Geometry: final body of the model. Coordinates: model frame, mm. Face numbers are marked on the shaded views. A direction names the side the tool comes from. Give positions to 0.01 mm unless a question says otherwise; leave off trailing zeros. Loops run counter-clockwise (first coordinate to the right, second up) from the corner with the lowest first, then second, coordinate; pieces in that order, holes last. Notation, with made-up numbers: (77.5, 44.5) -> (119.5, 44.5) arc R26 ccw to (119.5, 82.5) -> close; hole circle Ø7 at (23.5, 65). An arc over 180 degrees is marked (long way). Answer in a Markdown table with one row per item. Add a question column.
1) First-contact query: P1, Ø6, axis at x = -17.5, y = 18, coming from the +Z side; P2, Ø2, axis at y = -3, z = -0.5, coming from the +X side. Flat tips, straight axial feed; report the tip coordinate or a pass-through.
2) Section query D-D (x = 10). Return the cut outline in (y, z), plus the area to 3 significant figures.
3) Section query C-C (z = 1.25). Return the cut outline in (x, y).
4) Section query A-A (x = 0). Return the cut outline in (y, z).
5) Line query: line 1 (Z direction, x = 11, y = -19.5); line 2 (Z direction, x = 6.5, y = 1); line 3 (Y direction, x = 0, z = 2.5). Output: solid intervals per line, ascending. Write a range as from..to.
6) Access query for the marked faces 1 and 2. Directions: +Z, -Z, +X, -X, +Y, -Y. A direction counts if a zero-diameter tool reaches every point of the face in a straight line with its end or side. Return the directions, or none.
```python
from build123d import *

# Parameters (mm, degrees)
F0_R     = 25.4
F0_R_2   = 7.9375
F0_R_3   = 3.8735
F1_DEPTH = 1.5875
F2_DEPTH = 5.08
F3_SIZE  = 0.508
F4_DEPTH = 0.508


with BuildPart() as f1:
    # F0 (on Top) → F1 (new body)
    with BuildSketch(Plane.XY):
        Circle(F0_R)
        Circle(F0_R_2, mode=Mode.SUBTRACT)
        Circle(F0_R_2)
        Circle(F0_R_3, mode=Mode.SUBTRACT)
        Circle(F0_R_3)
    extrude(amount=-F1_DEPTH)

    # F0 (on Top) → F2 (join)
    with BuildSketch(Plane.XY):
        Circle(F0_R_3)
    extrude(amount=F2_DEPTH)

    # F3
    f3_edges = [f1.edges().sort_by_distance(p)[0] for p in [
        (-3.8735, 0, 5.08),
    ]]
    chamfer(f3_edges, length=F3_SIZE)

    # F0 (on Top) → F4 (join)
    with BuildSketch(Plane.XY):
        Circle(F0_R_2)
        Circle(F0_R_3, mode=Mode.SUBTRACT)
    extrude(amount=F4_DEPTH)


solid = f1.part
```
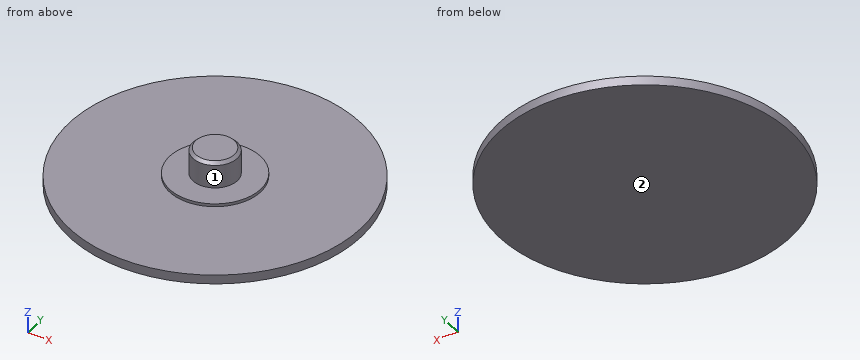
Evaluation:
| question | item | result |
|---|---|---|
| 1 | P1 | z = 0 |
| 1 | P2 | x = 25.32 |
| 2 | outline | (-23.35, -1.59) -> (23.35, -1.59) -> (23.35, 0) -> (-23.35, 0) -> close |
| 2 | area | 74.1 mm² |
| 3 | outline | circle Ø7.75 at (0, 0) |
| 4 | outline | (-25.4, -1.59) -> (25.4, -1.59) -> (25.4, 0) -> (7.94, 0) -> (7.94, 0.51) -> (3.87, 0.51) -> (3.87, 4.57) -> (3.37, 5.08) -> (-3.37, 5.08) -> (-3.87, 4.57) -> (-3.87, 0.51) -> (-7.94, 0.51) -> (-7.94, 0) -> (-25.4, 0) -> close |
| 5 | line 1 | -1.59..0 |
| 5 | line 2 | -1.59..0.51 |
| 5 | line 3 | -3.87..3.87 |
| 6 | face 1 | +Z |
| 6 | face 2 | -Z, +X, -X, +Y, -Y |
